Source: CAD feature listing. Evaluate the final solid. Frame: model axes, mm. A direction names the side the tool comes from. Give positions to 0.01 mm unless a question says otherwise; leave off trailing zeros. Loops run counter-clockwise (first coordinate to the right, second up) from the corner with the lowest first, then second, coordinate; pieces in that order, holes last. Notation, with made-up numbers: M -21.75,65.5 L 10.25,65.5 A22 ccw 10.25,101.5 Z; hole C 80,89.25 d9. An arc over 180 degrees is marked long. Answer in a Markdown table with one row per item.
Autodesk Inventor part; units mm, degrees
ref_plane "Work Plane1" through (15, 0, 0) normal (1, 0, 0) x (0, 0, -1)
ref_plane "YZ Plane" through (0, 0, 0) normal (1, 0, 0) x (0, 1, 0)
ref_plane "XZ Plane" through (0, 0, 0) normal (0, 1, 0) x (-1, 0, 0)
sketch "Sketch1" plane through (0, 0, 0) normal (1, 0, 0) x (0, 1, 0)
  circle A0 centre (0, 0) radius 2.925
  dimension "diameter" = 5.85
extrude "Shaft" add sketch "Sketch1" along normal mid plane 26
sketch "Sketch2" plane through (0, 0, 0) normal (0, 0, 1) x (1, 0, 0)
  line L0 (-13, -2.925) -> (-13, 2.925) construction
  line L1 (13, -2.925) -> (-13, -2.925) construction
  line L2 (13, 2.925) -> (13, -2.925) construction
  line L3 (-13, 2.925) -> (13, 2.925) construction
  line L4 (-13, -2.925) -> (13, -2.925)
  line L5 (-6, -2.925) -> (-6, -2.925)
  line L6 (-13, -2.925) -> (13, -2.925)
  line L7 (-11, 0) -> (-7, 0) construction
  line L8 (-10.1, -0.9) -> (-7.9, -0.9)
  line L9 (-7.9, 0.9) -> (-10.1, 0.9)
  arc A0 (-10.1, 0.9) -> (-10.1, -0.9) centre (-10.1, 0) ccw
  arc A1 (-7.9, -0.9) -> (-7.9, 0.9) centre (-7.9, 0) ccw
  point P0 (0, 0)
  point P1 (13, 0)
  point P2 (-9, 0)
  dimension "d17" = 1.8
  dimension "d20" = 2
  dimension "d21" = 1
  dimension "d22" = 7
extrude "Slot for Differential Gear" cut sketch "Sketch2" along normal through all both and the other way through all
ref_plane "Work Plane1" through (15, 0, 0) normal (1, 0, 0) x (0, 0, -1)
sketch "Sketch3" plane through (15, 0, 0) normal (1, 0, 0) x (0, 0, -1)
  arc A0 (1.6583, -2.5) -> (-1.6583, -2.5) centre (0, 0) ccw construction
  circle A1 centre (0, 0) radius 2.925 construction
  line L0 (-1.6583, -2.5) -> (1.6583, -2.5)
  arc A2 (1.6279, -2.4) -> (-1.6279, -2.4) centre (0, 0) ccw
  line L1 (1.6279, -2.4) -> (-1.6279, -2.4)
  point P0 (-1.5184, -2.5)
  point P1 (1.5184, -2.5)
  dimension "d49" = 3
  dimension "d50" = 2.5
  dimension "wheel_offset" = 0.1
extrude "Wheel Insert Profile" add sketch "Sketch3" along normal blind 12
loft "Loft1" add section 1 edges at (13, -2.925, 0) section 2 edges at (15, -2.4, 0) (15, 2.9, 0)
ref_plane "Work Plane2" through (11.5, 0, 0) normal (1, 0, 0) x (0, 0, -1)
sketch "Sketch4" plane through (11.5, 0, 0) normal (1, 0, 0) x (0, 0, -1)
  circle A0 centre (0, 0) radius 3.75
  dimension "d35" = 7.5
extrude "Stopper" add sketch "Sketch4" against normal blind 1
fillet "Fillet1" radius 0.5 2 edges at (11.5, 0, 3.75) (10.5, 0, 3.75)
sketch "Sketch8" plane through (-13, 0, 0) normal (-1, 0, 0) x (0, 0, 1)
  circle A0 centre (0, 0) radius 2.925
  circle A1 centre (0, 0) radius 2.7 construction
  circle A2 centre (0, 0) radius 2.65
  dimension "d68" = 5.4
  dimension "d69" = 0.05
extrude "Differential Gear Insert Profile" cut sketch "Sketch8" against normal blind 8
fillet "Fillet3" radius 1 1 edges at (-5, -2.925, 0)
chamfer "Chamfer4" distance 0.5 angle 45 2 edges at (-13, 0, -2.65) (27, 2.9, 0)
properties part number "rear shaft v2"
Q1. Contact query for flat-ended pins moving along their axis: pin 1 Ø1.1 at (x, z) = (-9, 1) entering from -Y; pin 2 Ø3.5 at (x, z) = (21, 1) entering from -Y; pin 3 Ø1.8 at (x, z) = (-9, -0.5) entering from +Y. Output: stop coordinate, or through.
Values follow:
| item | result |
|---|---|
| pin 1 | y = -2.61 |
| pin 2 | y = -2.4 |
| pin 3 | y = 2.65 |
Q2. Reachability of faces 5 (the cylindrical face through (-8.802, -2.351, 1.223)), 6 (the cylindrical face through (20.7, 2.9, 0.1)), 7 (the flat face through (27, 0, 0)), 8 (the cylindrical face through (-7, 0, 0)) from +Z, -Z, +X, -X, +Y, -Y: full face, straight path, thin tool, end or side. Return the list, or none.
Values follow:
| item | result |
|---|---|
| face 5 | -X |
| face 6 | +X |
| face 7 | +Z, -Z, +X, +Y, -Y |
| face 8 | +Z, -Z |
Q3. Section query A-A (x = -2.5). Output: boundary loops of the cut face in (y, z) (3 decimals), plus the area to 3 significant figures.
Values follow:
| item | result |
|---|---|
| outline | C 0,0 d5.85 |
| area | 26.9 mm^2 |
Q4. Ray query, probe 1 along Y at (x, z) = (-9, -2); probe 2 along X at (y, z) = (1.75, -2.5); probe 3 along Z at (x, y) = (-1, 0) (3 decimals). Return the intervals inside material, ascending. Write a range as from..to.
Values follow:
| item | result |
|---|---|
| probe 1 | -1.74..-0.9, 0.9..1.74 |
| probe 2 | 10.5..11.5 |
| probe 3 | -2.925..2.925 |
Q5. Mould query, pull axis Y, two halves, no side actions, for faces 1 (the flat face through (-13, 0, 0)), 2 (the cylindrical face through (-11, 0, 0)), 3 (the flat face through (21, -2.4, 0)), 4 (the cylindrical face through (12.24, -0.634, 2.855)). Classes: +Y half, -Y half, draft (parallel to the pull), parting line (faces both ways), or undercut.
Values follow:
| item | result |
|---|---|
| face 1 | draft |
| face 2 | undercut |
| face 3 | -Y half |
| face 4 | parting line |
